from build123d import *

# Parameters (mm, degrees)
SKETCH_1_W           = 153
SKETCH_1_H           = 97
EXTRUDE_1_DEPTH      = 2
SKETCH_2_W           = 30
SKETCH_2_H           = 56
EXTRUDE_2_DEPTH      = 2
EXTRUDE_3_DEPTH      = 2
SKETCH_4_W           = 10
SKETCH_4_H           = 42
SKETCH_4_R           = 2
EXTRUDE_4_DEPTH      = 2
SKETCH_6_R           = 2.25
CUT_EXTRUDE_1_DEPTH  = 2
SKETCH_7_W           = 50
SKETCH_7_H           = 56
CUT_EXTRUDE_2_DEPTH  = 2
SKETCH_8_W           = 48
SKETCH_8_H           = 62.484205033
CUT_EXTRUDE_3_DEPTH  = 2
FILLET_3_R           = 3
SKETCH_9_W           = 10
SKETCH_9_H           = 29.42018392
EXTRUDE_5_DEPTH      = 2
FILLET_4_R           = 3
SKETCH_10_W          = 18
SKETCH_10_H          = 20
CUT_EXTRUDE_4_DEPTH  = 2
FILLET_5_R           = 3
SKETCH_11_R          = 30
EXTRUDE_6_DEPTH      = 2
FILLET_6_R           = 3
SKETCH_12_R          = 1.25
CUT_EXTRUDE_5_DEPTH  = 2
SKETCH_13_R          = 1.5
CUT_EXTRUDE_6_DEPTH  = 10
SKETCH_14_R          = 1.5
CUT_EXTRUDE_7_DEPTH  = 10
CUT_EXTRUDE_8_DEPTH  = 10
FILLET_7_R           = 5
SKETCH_16_R          = 1.5
CUT_EXTRUDE_9_DEPTH  = 10
SKETCH_17_W          = 10
SKETCH_17_H          = 21
CUT_EXTRUDE_10_DEPTH = 10
FILLET_8_R           = 1
SKETCH_18_W          = 3
SKETCH_18_H          = 5
CUT_EXTRUDE_11_DEPTH = 10
FILLET_9_R           = 1
CUT_EXTRUDE_12_DEPTH = 2
FILLET_10_R          = 1
CUT_EXTRUDE_13_DEPTH = 2
FILLET_11_R          = 1


with BuildPart() as part:
    # 草图1 → 凸台-拉伸1 (new body)
    with BuildSketch(Plane(origin=(0, 0, 0), x_dir=(1, 0, 0), z_dir=(0, 1, 0))):
        Rectangle(SKETCH_1_W, SKETCH_1_H)
    extrude(amount=EXTRUDE_1_DEPTH)

    # 草图2 → 凸台-拉伸2 (add)
    with BuildSketch(Plane(origin=(0, 0, 0), x_dir=(1, 0, 0), z_dir=(0, 1, 0))):
        with Locations((0, 76.5)):
            Rectangle(SKETCH_2_W, SKETCH_2_H)
    extrude(amount=EXTRUDE_2_DEPTH)

    # 草图3 → 凸台-拉伸3 (add)
    with BuildSketch(Plane(origin=(0, 2, 0), x_dir=(1, 0, 0), z_dir=(0, 1, 0))):
        Polygon((-76.5, 48.5), (-15, 100.1), (-15, 48.5), align=None)
        Polygon((15, 100.1), (15, 48.5), (76.5, 48.5), align=None)
    extrude(amount=-EXTRUDE_3_DEPTH)

    # 草图4 → 凸台-拉伸4 (add)
    # profile 1 of 2: a face of its own
    with BuildSketch(Plane(origin=(0, 2, 0), x_dir=(1, 0, 0), z_dir=(0, 1, 0))):
        with Locations((-81.5, -27.5)):
            Rectangle(SKETCH_4_W, SKETCH_4_H)
        with Locations(Location((-81.5, -12.5, 0), (0, 0, 270))):
            Circle(SKETCH_4_R, mode=Mode.SUBTRACT)
        with Locations(Location((-81.5, -42.5, 0), (0, 0, 90))):
            Circle(SKETCH_4_R, mode=Mode.SUBTRACT)
    # profile 2 of 2: a face of its own
    with BuildSketch(Plane(origin=(0, 2, 0), x_dir=(1, 0, 0), z_dir=(0, 1, 0))):
        with Locations((81.5, -27.5)):
            Rectangle(SKETCH_4_W, SKETCH_4_H)
        with Locations(Location((81.5, -42.5, 0), (0, 0, 270))):
            Circle(SKETCH_4_R, mode=Mode.SUBTRACT)
        with Locations(Location((81.5, -12.5, 0), (0, 0, 90))):
            Circle(SKETCH_4_R, mode=Mode.SUBTRACT)
    extrude(amount=-EXTRUDE_4_DEPTH)

    # 草图6 → 切除-拉伸1 (cut)
    with BuildSketch(Plane(origin=(0, 2, 0), x_dir=(1, 0, 0), z_dir=(0, 1, 0))):
        with Locations(Location((14, 58.5, 0), (0, 0, 270))):
            Circle(SKETCH_6_R)
        with Locations(Location((-14, 58.5, 0), (0, 0, 90))):
            Circle(SKETCH_6_R)
    extrude(amount=-CUT_EXTRUDE_1_DEPTH, mode=Mode.SUBTRACT)

    # 草图7 → 切除-拉伸2 (cut)
    with BuildSketch(Plane(origin=(0, 2, 0), x_dir=(1, 0, 0), z_dir=(0, 1, 0))):
        with Locations((-46, -20.5)):
            Rectangle(SKETCH_7_W, SKETCH_7_H)
        with Locations((46, -20.5)):
            Rectangle(SKETCH_7_W, SKETCH_7_H)
    extrude(amount=-CUT_EXTRUDE_2_DEPTH, mode=Mode.SUBTRACT)

    # 草图8 → 切除-拉伸3 (cut)
    with BuildSketch(Plane(origin=(0, 2, 0), x_dir=(1, 0, 0), z_dir=(0, 1, 0))):
        with Locations((0, 93.742102517)):
            Rectangle(SKETCH_8_W, SKETCH_8_H)
    extrude(amount=-CUT_EXTRUDE_3_DEPTH, mode=Mode.SUBTRACT)

    # 圆角3
    fillet_3_edges = [part.edges().sort_by_distance(p)[0] for p in [
        (-21, 1, -7.5),
        (-21, 1, 48.5),
        (-71, 1, 48.5),
        (-71, 1, -7.5),
        (21, 1, -7.5),
        (71, 1, -7.5),
        (71, 1, 48.5),
        (21, 1, 48.5),
    ]]
    fillet(fillet_3_edges, radius=FILLET_3_R)

    # 草图9 → 凸台-拉伸5 (add)
    with BuildSketch(Plane(origin=(0, 2, 0), x_dir=(1, 0, 0), z_dir=(0, 1, 0))):
        with Locations((-81.5, 8.21009196)):
            Rectangle(SKETCH_9_W, SKETCH_9_H)
        with Locations((81.5, 8.21009196)):
            Rectangle(SKETCH_9_W, SKETCH_9_H)
    extrude(amount=-EXTRUDE_5_DEPTH)

    # 圆角4
    fillet_4_edges = [part.edges().sort_by_distance(p)[0] for p in [
        (-86.5, 1, -22.92018392),
        (-76.5, 1, -22.92018392),
    ]]
    fillet(fillet_4_edges, radius=FILLET_4_R)

    # 草图10 → 切除-拉伸4 (cut)
    with BuildSketch(Plane(origin=(0, 2, 0), x_dir=(1, 0, 0), z_dir=(0, 1, 0))):
        with Locations((0, 52.5)):
            Rectangle(SKETCH_10_W, SKETCH_10_H)
    extrude(amount=-CUT_EXTRUDE_4_DEPTH, mode=Mode.SUBTRACT)

    # 圆角5
    fillet_5_edges = [part.edges().sort_by_distance(p)[0] for p in [
        (24, 1, -92.548780488),
        (-24, 1, -92.548780488),
        (9, 1, -62.5),
        (9, 1, -42.5),
        (-9, 1, -42.5),
        (-9, 1, -62.5),
    ]]
    fillet(fillet_5_edges, radius=FILLET_5_R)

    # 草图11 → 凸台-拉伸6 (add)
    with BuildSketch(Plane(origin=(0, 2, 0), x_dir=(1, 0, 0), z_dir=(0, 1, 0))):
        with Locations((-36.5, 24.5)):
            Circle(SKETCH_11_R)
        with Locations((36.5, 24.5)):
            Circle(SKETCH_11_R)
    extrude(amount=-EXTRUDE_6_DEPTH)

    # 圆角6
    fillet_6_edges = [part.edges().sort_by_distance(p)[0] for p in [
        (86.5, 1, -22.92018392),
        (-86.5, 1, 48.5),
        (86.5, 1, 48.5),
    ]]
    fillet(fillet_6_edges, radius=FILLET_6_R)

    # 草图12 → 切除-拉伸5 (cut)
    with BuildSketch(Plane(origin=(0, 2, 0), x_dir=(1, 0, 0), z_dir=(0, 1, 0))):
        with Locations(Location((11, -12.5, 0), (0, 0, 270))):
            Circle(SKETCH_12_R)
        with Locations(Location((-15, -12.5, 0), (0, 0, 90))):
            Circle(SKETCH_12_R)
        with Locations(Location((-15, -38.5, 0), (0, 0, 270))):
            Circle(SKETCH_12_R)
    extrude(amount=-CUT_EXTRUDE_5_DEPTH, mode=Mode.SUBTRACT)

    # 草图13 → 切除-拉伸6 (cut)
    with BuildSketch(Plane(origin=(0, 2, 0), x_dir=(1, 0, 0), z_dir=(0, 1, 0))):
        with Locations(Location((-72, 46.5, 0), (0, 0, 270))):
            Circle(SKETCH_13_R)
        with Locations(Location((72, 46.5, 0), (0, 0, 270))):
            Circle(SKETCH_13_R)
    extrude(amount=-CUT_EXTRUDE_6_DEPTH, mode=Mode.SUBTRACT)

    # 草图14 → 切除-拉伸7 (cut)
    with BuildSketch(Plane(origin=(0, 2, 0), x_dir=(1, 0, 0), z_dir=(0, 1, 0))):
        with Locations(Location((-33.860465116, 78.5, 0), (0, 0, 270))):
            Circle(SKETCH_14_R)
        with Locations(Location((33.860465116, 78.5, 0), (0, 0, 270))):
            Circle(SKETCH_14_R)
    extrude(amount=-CUT_EXTRUDE_7_DEPTH, mode=Mode.SUBTRACT)

    # 草图15 → 切除-拉伸8 (cut)
    with BuildSketch(Plane(origin=(0, 2, 0), x_dir=(1, 0, 0), z_dir=(0, 1, 0))):
        with BuildLine():
            Line((21, -12.5), (21, -48.5))
            Line((21, -48.5), (-15, -48.5))
            ThreePointArc((-15, -48.5), (10.455844123, -37.955844123), (21, -12.5))
        make_face()
    extrude(amount=-CUT_EXTRUDE_8_DEPTH, mode=Mode.SUBTRACT)

    # 圆角7
    fillet_7_edges = [part.edges().sort_by_distance(p)[0] for p in [
        (-21, 1, 1.185599078),
        (21, 1, 1.185599078),
    ]]
    fillet(fillet_7_edges, radius=FILLET_7_R)

    # 草图16 → 切除-拉伸9 (cut)
    with BuildSketch(Plane(origin=(0, 2, 0), x_dir=(1, 0, 0), z_dir=(0, 1, 0))):
        with Locations(Location((9.5, 9.5, 0), (0, 0, 270))):
            Circle(SKETCH_16_R)
        with Locations(Location((-9.5, 9.5, 0), (0, 0, 270))):
            Circle(SKETCH_16_R)
    extrude(amount=-CUT_EXTRUDE_9_DEPTH, mode=Mode.SUBTRACT)

    # 草图17 → 切除-拉伸10 (cut)
    with BuildSketch(Plane(origin=(0, 2, 0), x_dir=(1, 0, 0), z_dir=(0, 1, 0))):
        with Locations((0, 12.5)):
            Rectangle(SKETCH_17_W, SKETCH_17_H)
    extrude(amount=-CUT_EXTRUDE_10_DEPTH, mode=Mode.SUBTRACT)

    # 圆角8
    fillet_8_edges = [part.edges().sort_by_distance(p)[0] for p in [
        (5, 1, -23),
        (5, 1, -2),
        (-5, 1, -2),
        (-5, 1, -23),
    ]]
    fillet(fillet_8_edges, radius=FILLET_8_R)

    # 草图18 → 切除-拉伸11 (cut)
    with BuildSketch(Plane(origin=(0, 2, 0), x_dir=(1, 0, 0), z_dir=(0, 1, 0))):
        with Locations((0, -0.5)):
            Rectangle(SKETCH_18_W, SKETCH_18_H)
    extrude(amount=-CUT_EXTRUDE_11_DEPTH, mode=Mode.SUBTRACT)

    # 圆角9
    fillet_9_edges = [part.edges().sort_by_distance(p)[0] for p in [
        (-1.5, 1, -2),
        (1.5, 1, -2),
        (1.5, 1, 3),
        (-1.5, 1, 3),
    ]]
    fillet(fillet_9_edges, radius=FILLET_9_R)

    # 草图19 → 切除-拉伸12 (cut)
    with BuildSketch(Plane(origin=(0, 2, 0), x_dir=(1, 0, 0), z_dir=(0, 1, 0))):
        Polygon((-13, -14.5), (-13, -33.671572875), (6.171572875, -14.5), align=None)
    extrude(amount=-CUT_EXTRUDE_12_DEPTH, mode=Mode.SUBTRACT)

    # 圆角10
    fillet_10_edges = [part.edges().sort_by_distance(p)[0] for p in [
        (-13, 1, 14.5),
        (6.171572875, 1, 14.5),
        (-13, 1, 33.671572875),
    ]]
    fillet(fillet_10_edges, radius=FILLET_10_R)

    # 草图21 → 切除-拉伸13 (cut)
    with BuildSketch(Plane(origin=(0, 2, 0), x_dir=(1, 0, 0), z_dir=(0, 1, 0))):
        with BuildLine():
            Line((15.354785216, -13.802069033), (-12.077894802, -41.234749051))
            ThreePointArc((-12.077894802, -41.234749051), (6.669497464, -32.549461299), (15.354785216, -13.802069033))
        make_face()
    extrude(amount=-CUT_EXTRUDE_13_DEPTH, mode=Mode.SUBTRACT)

    # 圆角11
    fillet_11_edges = [part.edges().sort_by_distance(p)[0] for p in [
        (15.354785216, 1, 13.802069033),
        (-12.077894802, 1, 41.234749051),
    ]]
    fillet(fillet_11_edges, radius=FILLET_11_R)


solid = part.part
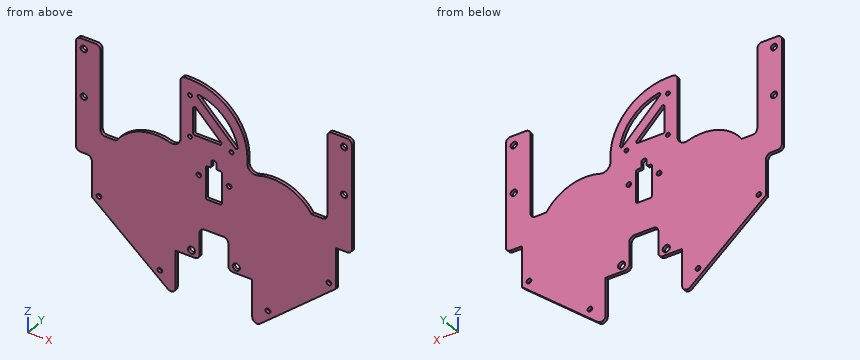
The model under review builds one solid part; all positions refer to its coordinate system, in mm. Coordinates: 2 decimals unless noted, no trailing zeros. Write each loop counter-clockwise with the first axis right and the second up, starting at its lowest first coordinate (ties: lowest second). Pieces come first, ordered by that corner, then holes. Notation, with made-up numbers: (77, 3) - (102, 3) arc R23 cw to (102, 26) - close; hole circle Ø5 at (-33, -19). An arc over 180 degrees is marked (long way). Answer as a JSON object with one key per item and string values. Group by question number.
1. Clearance check with flat-ended pins moving along their axes: pin 1 Ø0.6 at (x, y) = (-17, 1) entering from -Z; pin 2 Ø1.2 at (x, y) = (-3.5, 1) entering from -Z; pin 3 Ø1 at (y, z) = (1, -33.5) entering from -X. State where each tip first meets the part, or that it passes through.
2. To check wall thickness, follow probe 1 along X at (y, z) = (1.4, -46.5); probe 2 along X at (y, z) = (1.1, -18); probe 3 along X at (y, z) = (0.85, 42.5). State the ranges of each line that lie inside material, in increasing order.
3. Add section C-C (y = 0.4). Give the number of separate pieces and of enclosed holes in the cut face, plus the area to 3 significant figures.
4. Add section A-A (x = -81.5). Give the boundary of the cut face in (y, z).
5. Add section B-B (z = 34.5). Give the boundary of the cut face in (x, y).
Findings:
{
 "1": {"pin 1": "z = -62.5", "pin 2": "z = -42.5", "pin 3": "x = -76.5"},
 "2": {"probe 1": "-76.5 to -73.5, -70.5 to -9, 9 to 70.5, 73.5 to 76.5", "probe 2": "-86.5 to -5, 5 to 86.5", "probe 3": "-86.5 to -83.5, -79.5 to -71, -21 to 4.9, 71 to 79.5, 83.5 to 86.5"},
 "3": {"separate pieces": "1", "enclosed holes": "18", "area": "13,100 mm²"},
 "4": {"outline": "(0, -22.92) - (2, -22.92) - (2, 10.5) - (0, 10.5) - close; (0, 14.5) - (2, 14.5) - (2, 40.5) - (0, 40.5) - close; (0, 44.5) - (2, 44.5) - (2, 48.5) - (0, 48.5) - close"},
 "5": {"outline": "(-86.5, 0) - (-71, 0) - (-71, 2) - (-86.5, 2) - close; (-21, 0) - (-5.34, 0) - (-5.34, 2) - (-21, 2) - close; (4.52, 0) - (13.5, 0) - (13.5, 2) - (4.52, 2) - close; (71, 0) - (86.5, 0) - (86.5, 2) - (71, 2) - close"}
}
